The model under review builds one solid part; all positions refer to its coordinate system, in mm. A direction names the side the tool comes from. Coordinates: 2 decimals unless noted, no trailing zeros. Order: outer loops, then holes, each group sorted by start corner. A loop starts at its lowest first (then second) coordinate and runs counter-clockwise, first axis right, second up.
```python
from build123d import *

# Parameters (mm, degrees)
SKETCH_1_W      = 30
SKETCH_1_H      = 30
EXTRUDE_1_DEPTH = 3
EXTRUDE_START   = -3
SKETCH_2_W      = 25
SKETCH_2_H      = 5
EXTRUDE_2_DEPTH = 100
FILLET_1_R      = 5


with BuildPart() as part:
    # 草图1 → 凸台-拉伸1 (new body)
    # profile 1 of 3: a face of its own
    with BuildSketch(Plane.XY):
        Rectangle(SKETCH_1_W, SKETCH_1_H)
        with BuildLine():
            Line((-11.75, -10), (-11.75, 10))
            ThreePointArc((-11.75, 10), (-10, 11.75), (-8.25, 10))
            Line((-8.25, 10), (-8.25, -10))
            ThreePointArc((-8.25, -10), (-10, -11.75), (-11.75, -10))
        make_face(mode=Mode.SUBTRACT)
        with BuildLine():
            ThreePointArc((8.25, 10), (10, 11.75), (11.75, 10))
            Line((11.75, 10), (11.75, -10))
            ThreePointArc((11.75, -10), (10, -11.75), (8.25, -10))
            Line((8.25, -10), (8.25, 10))
        make_face(mode=Mode.SUBTRACT)
    # profile 2 of 3: a face of its own
    with BuildSketch(Plane.XY):
        Polygon((-55, -3), (-15, 15), (-15, -15), (-90, -30), (-115, -30), (-115, -15), align=None)
    # profile 3 of 3: a face of its own
    with BuildSketch(Plane.XY):
        Polygon((15, 15), (15, -15), (90, -30), (115, -30), (115, -15), (55, -3), align=None)
    extrude(amount=EXTRUDE_1_DEPTH)

    # 草图2 → 凸台-拉伸2 (add)
    with BuildSketch(Plane(origin=(0, 0, 0), x_dir=(-1, 0, 0), z_dir=(0, 0, -1)).offset(EXTRUDE_START)):
        with Locations((-102.5, -27.5)):
            Rectangle(SKETCH_2_W, SKETCH_2_H)
        with Locations((102.5, -27.5)):
            Rectangle(SKETCH_2_W, SKETCH_2_H)
    extrude(amount=-EXTRUDE_2_DEPTH)

    # 圆角1
    fillet_1_edges = [part.edges().sort_by_distance(p)[0] for p in [
        (102.5, -25, 3),
        (-102.5, -25, 3),
    ]]
    fillet(fillet_1_edges, radius=FILLET_1_R)


solid = part.part
```
(1) We need section C-C, the plane x = 61.5. Write out the cut boundary in (y, z).
A:
outline: (-24.3, 0) - (-4.3, 0) - (-4.3, 3) - (-24.3, 3) - close
(2) For pin 1 Ø2.5 at (x, z) = (1.5, 1) entering from -Y; pin 2 Ø12.5 at (x, z) = (-104, 52.5) entering from +Y; pin 3 Ø3.5 at (y, z) = (-1, 2) entering from +X, all flat-tipped, find the tip position at first contact; note any pin that passes through.
A:
pin 1: stops at y = -15
pin 2: stops at y = -25
pin 3: stops at x = 54.44
(3) Machinability: for faces 5 (the face through (103, -30, 51)), 6 (the face through (90, -27, 52)), 7 (the face through (-115, -27, 47)), 8 (the face through (52, -22.4, 1.5)), 9 (the face through (-102, -25, 55)), which of the approach directions +Z, -Z, +X, -X, +Y, -Y give a long, thin tool a straight path to every point of the face, cutting with its end or side? Answer none if there is none.
A:
face 5: +Z, -Z, +X, -X, -Y
face 6: +Z, +Y, -Y
face 7: +Z, -Z, -X, +Y, -Y
face 8: +Z, -Z, -Y
face 9: +Z, +X, -X, +Y
(4) We need section B-B, the plane y = 4.5. Write out the cut boundary in (x, z).
A:
outline: (-38.33, 0) - (-11.75, 0) - (-11.75, 3) - (-38.33, 3) - close; (-8.25, 0) - (8.25, 0) - (8.25, 3) - (-8.25, 3) - close; (11.75, 0) - (38.33, 0) - (38.33, 3) - (11.75, 3) - close
(5) Draft analysis for pull direction X (two halves, no side actions). For faces 1 (the face through (-35, 6, 1)), 2 (the face through (115, -27, 47)), 3 (the face through (-52, -22.4, 1.5)), 4 (the face through (103, -27, 103)), state which applies: released by +X, released by -X, zero draft, split by the parting line, or undercut.
A:
face 1: released by -X
face 2: released by +X
face 3: undercut
face 4: zero draft
(6) We need section A-A, the plane z = 43.5. Write out the cut boundary in (x, y), and give its area (3 significant figures).
A:
outline: (-115, -30) - (-90, -30) - (-90, -25) - (-115, -25) - close; (90, -30) - (115, -30) - (115, -25) - (90, -25) - close
area: 250 mm2
(7) We need section D-D, the plane x = -48. Write out the cut boundary in (y, z).
A:
outline: (-21.6, 0) - (0.15, 0) - (0.15, 3) - (-21.6, 3) - close
(8) Wall thickness on probe 1 along Z at (x, y) = (-69.5, -24.5); probe 2 along Y at (x, z) = (99, 18.5): over which ranges is each line inside the solid? List them lowest first.
A:
probe 1: z = 0 to 3
probe 2: y = -30 to -25
